Read the model definition and answer for the solid it produces. Units are mm, in the model's axes. Face numbers are marked on the shaded views. A direction names the side the tool comes from. Coordinates: 2 decimals unless noted, no trailing zeros. Loops run counter-clockwise (first coordinate to the right, second up) from the corner with the lowest first, then second, coordinate; pieces in that order, holes last. Notation, with made-up numbers: (19, 22) - (63, 22) arc R17 ccw to (63, 34) - close; hole circle Ø6 at (60, 20). An arc over 180 degrees is marked (long way). Use one line per item in the form item = value.
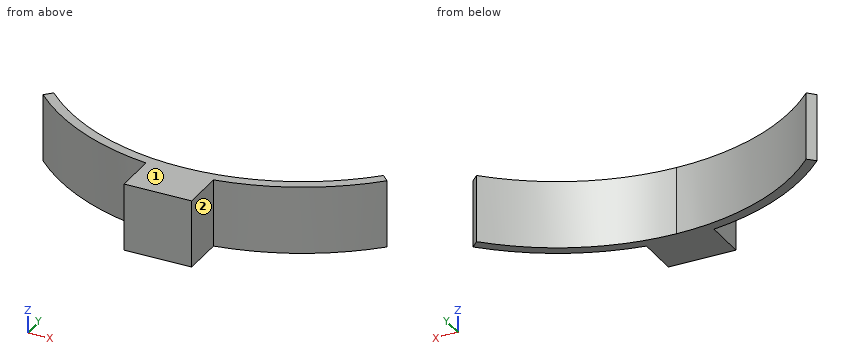
from build123d import *

# Parameters (mm, degrees)
F1_DEPTH = 20


with BuildPart() as f1:
    # F0 (on Top) → F1 (new body)
    with BuildSketch(Plane.XY):
        with BuildLine():
            Line((0, -69), (10, -69))
            Line((10, -69), (10, -71.302174))
            ThreePointArc((10, -71.302174), (32.116996, -64.439883), (50.911688, -50.911688))
            Line((50.911688, -50.911688), (48.790368, -48.790368))
            ThreePointArc((48.790368, -48.790368), (26.405157, -63.747688), (0, -69))
        make_face()
        Polygon((10, -71.302174), (10, -69), (0, -69), (-10, -69), (-10, -71.302174), (-10, -84), (10, -84), align=None)
        with BuildLine():
            Line((-10, -69), (0, -69))
            ThreePointArc((0, -69), (-26.405157, -63.747688), (-48.790368, -48.790368))
            Line((-48.790368, -48.790368), (-50.911688, -50.911688))
            ThreePointArc((-50.911688, -50.911688), (-32.116996, -64.439883), (-10, -71.302174))
            Line((-10, -71.302174), (-10, -69))
        make_face()
    extrude(amount=F1_DEPTH)


solid = f1.part
Item 1: Find the intervals of material crossed by L1, parallel to X at y = -75.5, z = 11.25; L2, parallel to X at y = -57.5, z = 12.5; L3, parallel to X at y = -54.5, z = 8, in increasing order.
Results below:
L1 = -10 to 10
L2 = -43.33 to -38.14, 38.14 to 43.33
L3 = -47.05 to -42.32, 42.32 to 47.05
Item 2: The part is cut by section D-D on y = -81. Give the vertices of the cut face in (x, z), plus the area to 3 significant figures.
Results below:
outline = (-10, 0) - (10, 0) - (10, 20) - (-10, 20) - close
area = 400 mm²
Item 3: Which of the six approach directions +Z, -Z, +X, -X, +Y, -Y give full straight-line access (tool end or side, diameter ignored) to the marked faces 1 and 2?
Results below:
face_1 = +Z, +X, -X, +Y, -Y
face_2 = +Z, -Z, +X, -Y
Item 4: Each of these flat-tipped pins is pushed along its axis until it touches: P1, Ø10, axis at y = -66.5, z = 2, coming from the -X side; P2, Ø6, axis at y = -60, z = 2, coming from the -X side; P3, Ø5, axis at y = -69, z = 10, coming from the +X side. Where does it stop, or does it pass through?
Results below:
P1 = -37.44
P2 = -43.99
P3 = 27.6
Item 5: The part is cut by section A-A on y = -57. Give the vertices of the cut face in (x, z), plus the area to 3 significant figures.
Results below:
outline = (-43.99, 0) - (-38.88, 0) - (-38.88, 20) - (-43.99, 20) - close; (38.88, 0) - (43.99, 0) - (43.99, 20) - (38.88, 20) - close
area = 204 mm²
Item 6: The part is cut by section C-C on y = -62.5. Give the vertices of the cut face in (x, z).
Results below:
outline = (-35.75, 0) - (-29.24, 0) - (-29.24, 20) - (-35.75, 20) - close; (29.24, 0) - (35.75, 0) - (35.75, 20) - (29.24, 20) - close
Item 7: The part is cut by section B-B on z = 14. Give the vertices of the cut face in (x, y), plus the area to 3 significant figures.
Results below:
outline = (-50.91, -50.91) arc R72 ccw to (-10, -71.3) - (-10, -84) - (10, -84) - (10, -71.3) arc R72 ccw to (50.91, -50.91) - (48.79, -48.79) arc R69 cw to (0, -69) arc R69 cw to (-48.79, -48.79) - close
area = 577 mm²
